Check sheet for the modelled part. Datum: model origin and axes. Units: mm. A direction names the side the tool comes from. Round coordinates to 2 decimals unless told otherwise and drop trailing zeros. Write each loop counter-clockwise with the first axis right and the second up, starting at its lowest first coordinate (ties: lowest second). Pieces come first, ordered by that corner, then holes. Notation, with made-up numbers: (12.25, -8) -> (45.25, -8) arc R16 cw to (45.25, 5) -> close; hole circle Ø2 at (55.5, 64.25). An arc over 180 degrees is marked (long way). One line per item, written item: value.
from build123d import *

# Parameters (mm, degrees)
SKETCH1_R           = 2.65
BOSS_EXTRUDE1_DEPTH = 1
BOSS_EXTRUDE4_DEPTH = 4.5
BOSS_EXTRUDE5_DEPTH = 4.5


with BuildPart() as part:
    # Sketch1 → Boss-Extrude1 (new, symmetric)
    with BuildSketch(Plane(origin=(0, 0, 0), x_dir=(1, 0, 0), z_dir=(0, 1, 0))):
        with BuildLine():
            Line((4.5, 47.5), (-4.5, 47.5))
            Line((-4.5, 47.5), (-4.5, 44.5))
            Line((-4.5, 44.5), (-10.429017764, 32.931184851))
            ThreePointArc((-10.429017764, 32.931184851), (-12.17849868, 31.444109042), (-14.467089888, 31.629657472))
            Line((-14.467089888, 31.629657472), (-22.327869159, 35.658306849))
            ThreePointArc((-22.327869159, 35.658306849), (-29.057989367, 33.48909455), (-26.888777069, 26.758974343))
            Line((-26.888777069, 26.758974343), (-19.027997797, 22.730324967))
            ThreePointArc((-19.027997797, 22.730324967), (-17.540921988, 20.980844051), (-17.726470418, 18.692252842))
            Line((-17.726470418, 18.692252842), (-19.726418437, 14.789915246))
            Line((-19.726418437, 14.789915246), (-25, 4.5))
            Line((-25, 4.5), (-25, -4.5))
            Line((-25, -4.5), (-19.726418437, -14.789915246))
            Line((-19.726418437, -14.789915246), (-17.726470418, -18.692252842))
            ThreePointArc((-17.726470418, -18.692252842), (-17.540921988, -20.980844051), (-19.027997797, -22.730324967))
            Line((-19.027997797, -22.730324967), (-26.888777069, -26.758974343))
            ThreePointArc((-26.888777069, -26.758974343), (-29.057989367, -33.48909455), (-22.327869159, -35.658306849))
            Line((-22.327869159, -35.658306849), (-14.467089888, -31.629657472))
            ThreePointArc((-14.467089888, -31.629657472), (-12.17849868, -31.444109042), (-10.429017764, -32.931184851))
            Line((-10.429017764, -32.931184851), (-4.5, -44.5))
            Line((-4.5, -44.5), (-4.5, -47.5))
            Line((-4.5, -47.5), (4.5, -47.5))
            Line((4.5, -47.5), (4.5, -44.5))
            Line((4.5, -44.5), (10.429017764, -32.931184851))
            ThreePointArc((10.429017764, -32.931184851), (12.17849868, -31.444109042), (14.467089888, -31.629657472))
            Line((14.467089888, -31.629657472), (22.327869159, -35.658306849))
            ThreePointArc((22.327869159, -35.658306849), (29.057989367, -33.48909455), (26.888777069, -26.758974343))
            Line((26.888777069, -26.758974343), (19.027997797, -22.730324967))
            ThreePointArc((19.027997797, -22.730324967), (17.540921988, -20.980844051), (17.726470418, -18.692252842))
            Line((17.726470418, -18.692252842), (19.726418437, -14.789915246))
            Line((19.726418437, -14.789915246), (25, -4.5))
            Line((25, -4.5), (25, 4.5))
            Line((25, 4.5), (19.726418437, 14.789915246))
            Line((19.726418437, 14.789915246), (17.726470418, 18.692252842))
            ThreePointArc((17.726470418, 18.692252842), (17.540921988, 20.980844051), (19.027997797, 22.730324967))
            Line((19.027997797, 22.730324967), (26.888777069, 26.758974343))
            ThreePointArc((26.888777069, 26.758974343), (29.057989367, 33.48909455), (22.327869159, 35.658306849))
            Line((22.327869159, 35.658306849), (14.467089888, 31.629657472))
            ThreePointArc((14.467089888, 31.629657472), (12.17849868, 31.444109042), (10.429017764, 32.931184851))
            Line((10.429017764, 32.931184851), (4.5, 44.5))
            Line((4.5, 44.5), (4.5, 47.5))
        make_face()
        with Locations(Location((-22.25, 30, 0), (0, 0, 270))):
            Circle(SKETCH1_R, mode=Mode.SUBTRACT)
        with Locations(Location((-22.25, -30, 0), (0, 0, 270))):
            Circle(SKETCH1_R, mode=Mode.SUBTRACT)
        with Locations(Location((22.25, 30, 0), (0, 0, 270))):
            Circle(SKETCH1_R, mode=Mode.SUBTRACT)
        with Locations(Location((22.25, -30, 0), (0, 0, 270))):
            Circle(SKETCH1_R, mode=Mode.SUBTRACT)
        with BuildLine():
            Line((-4, 34.512880186), (-12.184076307, 18.543950806))
            ThreePointArc((-12.184076307, 18.543950806), (-11.245300372, 13.197591441), (-16.133581658, 10.837598902))
            Line((-16.133581658, 10.837598902), (-19.637851096, 4))
            Line((-19.637851096, 4), (-4, 4))
            Line((-4, 4), (-4, 34.512880186))
        make_face(mode=Mode.SUBTRACT)
        with BuildLine():
            Line((4, 4), (4, 34.512880186))
            Line((4, 34.512880186), (12.184076307, 18.543950806))
            ThreePointArc((12.184076307, 18.543950806), (11.245300372, 13.197591441), (16.133581658, 10.837598902))
            Line((16.133581658, 10.837598902), (19.637851096, 4))
            Line((19.637851096, 4), (4, 4))
        make_face(mode=Mode.SUBTRACT)
        with BuildLine():
            Line((4, -34.512880186), (12.184076307, -18.543950806))
            ThreePointArc((12.184076307, -18.543950806), (11.245300372, -13.197591441), (16.133581658, -10.837598902))
            Line((16.133581658, -10.837598902), (19.637851096, -4))
            Line((19.637851096, -4), (4, -4))
            Line((4, -4), (4, -34.512880186))
        make_face(mode=Mode.SUBTRACT)
        with BuildLine():
            Line((-4, -4), (-4, -34.512880186))
            Line((-4, -34.512880186), (-12.184076307, -18.543950806))
            ThreePointArc((-12.184076307, -18.543950806), (-11.245300372, -13.197591441), (-16.133581658, -10.837598902))
            Line((-16.133581658, -10.837598902), (-19.637851096, -4))
            Line((-19.637851096, -4), (-4, -4))
        make_face(mode=Mode.SUBTRACT)
    extrude(amount=BOSS_EXTRUDE1_DEPTH, both=True)

    # Sketch6 → Boss-Extrude4 (add, symmetric)
    with BuildSketch(Plane(origin=(0, 0, 0), x_dir=(0, 0, -1), z_dir=(1, 0, 0))):
        Polygon((47.5, 1), (47.5, 6), (44.5, 6), (45.5, 5), (45.5, 1), align=None)
        Polygon((-45.5, 1), (-47.5, 1), (-47.5, 6), (-44.5, 6), (-45.5, 5), align=None)
    extrude(amount=BOSS_EXTRUDE4_DEPTH, both=True)

    # Sketch4 → Boss-Extrude5 (add, symmetric)
    with BuildSketch(Plane.XY):
        Polygon((30, 10.5), (30, 15.5), (27, 15.5), (28, 14.5), (28, 10.5), (26.728712295, 10.5), (22.598277512, 1), (25, 1), (25, -1), align=None)
        Polygon((-28, 14.5), (-28, 10.5), (-26.728712295, 10.5), (-22.598277512, 1), (-25, 1), (-25, -1), (-30, 10.5), (-30, 15.5), (-27, 15.5), align=None)
    extrude(amount=BOSS_EXTRUDE5_DEPTH, both=True)


solid = part.part
Item 1: Release check for a two-part mould opening along X. For faces 5 (the flat face through (4.5, 3, -46)), 6 (the flat face through (0, 6, 46)), 7 (the flat face through (17.86, -0.01, 7.47)), 8 (the flat face through (-27.465, 4.67, 0.063)) record: pulls with the +X half, pulls with the -X half, needs draft (parallel to the pull), parting line crosses it, or undercut.
Result set:
face 5: pulls with the +X half
face 6: needs draft
face 7: undercut
face 8: pulls with the -X half
Item 2: Sectioned sample at A-A (z = -30). Enter the section's corners in (x, y), then the cut area to 3 significant figures.
Result set:
outline: (-29.46, -1) -> (-24.9, -1) -> (-24.9, 1) -> (-29.46, 1) -> close; (-19.6, -1) -> (-6.31, -1) -> (-6.31, 1) -> (-19.6, 1) -> close; (-4, -1) -> (4, -1) -> (4, 1) -> (-4, 1) -> close; (6.31, -1) -> (19.6, -1) -> (19.6, 1) -> (6.31, 1) -> close; (24.9, -1) -> (29.46, -1) -> (29.46, 1) -> (24.9, 1) -> close
area: 87.4 mm^2
Item 3: Tool access check on faces 1 (the flat face through (-18.45, 0.01, 33.67)), 2 (the flat face through (4.5, 3, 46)), 3 (the flat face through (-12, 0, -4)), 4 (the flat face through (23.01, 0.01, 24.77)). Record the directions out of +Z, -Z, +X, -X, +Y, -Y that give a thin tool (end or side, any length) a straight path to the whole face; none if there is none.
Result set:
face 1: +Z, +Y, -Y
face 2: +Z, +X, +Y, -Y
face 3: +Y, -Y
face 4: +X, +Y, -Y
Item 4: Material ranges on line 1 along X through (y, z) = (0, -30); line 2 along Z through (x, y) = (21, 0.5); line 3 along Y through (x, z) = (-21, -2.5), recorded low to high.
Result set:
line 1: -29.46 to -24.9, -19.6 to -6.31, -4 to 4, 6.31 to 19.6, 24.9 to 29.46
line 2: -34.98 to -32.34, -27.66 to -23.74, -12.3 to 12.3, 23.74 to 27.66, 32.34 to 34.98
line 3: -1 to 1
Item 5: Sectioned sample at C-C (z = 13). Enter the section's corners in (x, y), then the cut area to 3 significant figures.
Result set:
outline: (-20.64, -1) -> (-11.35, -1) -> (-11.35, 1) -> (-20.64, 1) -> close; (-4, -1) -> (4, -1) -> (4, 1) -> (-4, 1) -> close; (11.35, -1) -> (20.64, -1) -> (20.64, 1) -> (11.35, 1) -> close
area: 53.2 mm^2
Item 6: Depth check by flat-ended pin: pin 1 (10 mm diameter, centred on x = 12.5, z = 17, fed in from +Y); pin 2 (1.6 mm diameter, centred on x = -15, y = 0, fed in from -Z); pin 3 (1 mm diameter, centred on x = 11.5, y = 0, fed in from -Z); pin 4 (5 mm diameter, centred on x = 20.5, z = -31.5, fed in from -Y). Enter the tip coordinate at first touch or a pass-through.
Result set:
pin 1: y = 1
pin 2: z = -32.31
pin 3: z = -32.16
pin 4: y = -1
Item 7: Sectioned sample at D-D (x = -7). Enter the section's corners in (y, z), then the cut area to 3 significant figures.
Result set:
outline: (-1, -39.62) -> (1, -39.62) -> (1, -28.66) -> (-1, -28.66) -> close; (-1, -4) -> (1, -4) -> (1, 4) -> (-1, 4) -> close; (-1, 28.66) -> (1, 28.66) -> (1, 39.62) -> (-1, 39.62) -> close
area: 59.9 mm^2
Item 8: Sectioned sample at B-B (y = 3.5). Enter the section's corners in (x, z).
Result set:
outline: (-26.96, -4.5) -> (-23.69, -4.5) -> (-23.69, 4.5) -> (-26.96, 4.5) -> close; (-4.5, -47.5) -> (4.5, -47.5) -> (4.5, -45.5) -> (-4.5, -45.5) -> close; (-4.5, 45.5) -> (4.5, 45.5) -> (4.5, 47.5) -> (-4.5, 47.5) -> close; (23.69, -4.5) -> (26.96, -4.5) -> (26.96, 4.5) -> (23.69, 4.5) -> close
